```python
from build123d import *

# Parameters (mm, degrees)
SKETCH_1_W          = 300
SKETCH_1_H          = 300
EXTRUDE_1_DEPTH     = 5
SKETCH_2_R          = 1.6
CUT_EXTRUDE_1_DEPTH = 5
SKETCH_3_W          = 20
SKETCH_3_H          = 50
EXTRUDE_2_DEPTH     = 5
SKETCH_5_R          = 1.6
CUT_EXTRUDE_2_DEPTH = 462.004338374
CHAMFER_1_SIZE      = 20
FILLET_1_R          = 20
FILLET_2_R          = 5
FILLET_3_R          = 10


with BuildPart() as part:
    # 草图1 → 凸台-拉伸1 (new body)
    with BuildSketch(Plane.XY):
        with Locations((150, 150)):
            Rectangle(SKETCH_1_W, SKETCH_1_H)
    extrude(amount=EXTRUDE_1_DEPTH)

    # 草图2 → 切除-拉伸1 (cut)
    with BuildSketch(Plane.XY.offset(5)):
        with Locations((10, 10)):
            Circle(SKETCH_2_R)
        with Locations((290, 10)):
            Circle(SKETCH_2_R)
        with Locations((290, 290)):
            Circle(SKETCH_2_R)
        with Locations((10, 290)):
            Circle(SKETCH_2_R)
        with Locations((10, 270)):
            Circle(SKETCH_2_R)
        with Locations((10, 250)):
            Circle(SKETCH_2_R)
        with Locations((10, 30)):
            Circle(SKETCH_2_R)
        with Locations((10, 50)):
            Circle(SKETCH_2_R)
        with Locations((30, 290)):
            Circle(SKETCH_2_R)
        with Locations((50, 290)):
            Circle(SKETCH_2_R)
        with Locations((270, 290)):
            Circle(SKETCH_2_R)
        with Locations((250, 290)):
            Circle(SKETCH_2_R)
        with Locations((290, 270)):
            Circle(SKETCH_2_R)
        with Locations((290, 250)):
            Circle(SKETCH_2_R)
        with Locations((290, 30)):
            Circle(SKETCH_2_R)
        with Locations((290, 50)):
            Circle(SKETCH_2_R)
        with Locations((270, 10)):
            Circle(SKETCH_2_R)
        with Locations((250, 10)):
            Circle(SKETCH_2_R)
        with Locations((30, 10)):
            Circle(SKETCH_2_R)
        with Locations((50, 10)):
            Circle(SKETCH_2_R)
    extrude(amount=-CUT_EXTRUDE_1_DEPTH, mode=Mode.SUBTRACT)

    # 草图3 → 凸台-拉伸2 (add, through all)
    with BuildSketch(Plane.XY.offset(5)):
        with Locations((80, -25)):
            Rectangle(SKETCH_3_W, SKETCH_3_H)
        with Locations((80, 325)):
            Rectangle(SKETCH_3_W, SKETCH_3_H)
        with Locations((220, 325)):
            Rectangle(SKETCH_3_W, SKETCH_3_H)
        with Locations((220, -25)):
            Rectangle(SKETCH_3_W, SKETCH_3_H)
    extrude(amount=-EXTRUDE_2_DEPTH)

    # 草图5 → 切除-拉伸2 (cut, through all)
    with BuildSketch(Plane.XY.offset(5)):
        with Locations((80, 345)):
            Circle(SKETCH_5_R)
        with Locations((80, 325)):
            Circle(SKETCH_5_R)
        with Locations((80, 305)):
            Circle(SKETCH_5_R)
        with Locations((80, 255)):
            Circle(SKETCH_5_R)
        with Locations((80, 275)):
            Circle(SKETCH_5_R)
        with Locations(Location((80, 25, 0), (0, 0, 180))):
            Circle(SKETCH_5_R)
        with Locations(Location((80, 45, 0), (0, 0, 180))):
            Circle(SKETCH_5_R)
        with Locations(Location((80, -5, 0), (0, 0, 180))):
            Circle(SKETCH_5_R)
        with Locations(Location((80, -25, 0), (0, 0, 180))):
            Circle(SKETCH_5_R)
        with Locations(Location((80, -45, 0), (0, 0, 180))):
            Circle(SKETCH_5_R)
        with Locations((220, -45)):
            Circle(SKETCH_5_R)
        with Locations((220, -25)):
            Circle(SKETCH_5_R)
        with Locations((220, -5)):
            Circle(SKETCH_5_R)
        with Locations((220, 45)):
            Circle(SKETCH_5_R)
        with Locations((220, 25)):
            Circle(SKETCH_5_R)
        with Locations(Location((220, 275, 0), (0, 0, 180))):
            Circle(SKETCH_5_R)
        with Locations(Location((220, 255, 0), (0, 0, 180))):
            Circle(SKETCH_5_R)
        with Locations(Location((220, 305, 0), (0, 0, 180))):
            Circle(SKETCH_5_R)
        with Locations(Location((220, 325, 0), (0, 0, 180))):
            Circle(SKETCH_5_R)
        with Locations(Location((220, 345, 0), (0, 0, 180))):
            Circle(SKETCH_5_R)
    extrude(amount=-CUT_EXTRUDE_2_DEPTH, mode=Mode.SUBTRACT)

    # 倒角1
    chamfer_1_edges = [part.edges().sort_by_distance(p)[0] for p in [
        (210, 0, 2.5),
        (230, 0, 2.5),
        (230, 300, 2.5),
        (210, 300, 2.5),
        (90, 300, 2.5),
        (70, 300, 2.5),
        (70, 0, 2.5),
        (90, 0, 2.5),
    ]]
    chamfer(chamfer_1_edges, length=CHAMFER_1_SIZE)

    # 圆角1
    fillet_1_edges = [part.edges().sort_by_distance(p)[0] for p in [
        (230, -20, 2.5),
        (250, 0, 2.5),
        (110, 0, 2.5),
        (190, 0, 2.5),
        (210, -20, 2.5),
        (90, -20, 2.5),
        (50, 0, 2.5),
        (70, -20, 2.5),
        (250, 300, 2.5),
        (230, 320, 2.5),
        (210, 320, 2.5),
        (110, 300, 2.5),
        (190, 300, 2.5),
        (90, 320, 2.5),
        (70, 320, 2.5),
        (50, 300, 2.5),
    ]]
    fillet(fillet_1_edges, radius=FILLET_1_R)

    # 圆角2
    fillet_2_edges = [part.edges().sort_by_distance(p)[0] for p in [
        (230, -50, 2.5),
        (210, -50, 2.5),
        (230, 350, 2.5),
        (210, 350, 2.5),
        (70, 350, 2.5),
        (90, 350, 2.5),
        (70, -50, 2.5),
        (90, -50, 2.5),
    ]]
    fillet(fillet_2_edges, radius=FILLET_2_R)

    # 圆角3
    fillet_3_edges = [part.edges().sort_by_distance(p)[0] for p in [
        (0, 300, 2.5),
        (300, 300, 2.5),
        (300, 0, 2.5),
        (0, 0, 2.5),
    ]]
    fillet(fillet_3_edges, radius=FILLET_3_R)


solid = part.part
```
Check sheet for the modelled part. Datum: model origin and axes. Units: mm. A direction names the side the tool comes from. Round coordinates to 2 decimals unless told otherwise and drop trailing zeros. Order: outer loops, then holes, each group sorted by start corner. A loop starts at its lowest first (then second) coordinate and runs counter-clockwise, first axis right, second up.
1) Mould release check, pull along X, two halves, no side actions. Record for faces 1 (the flat face through (240, 310, 3)), 2 (the flat face through (60, 310, 3)), 3 (the flat face through (100, -10, 3)): +X half, -X half, draft (parallel to the pull), parting line (faces both ways), or undercut.
2) Section check A-A (z = 2.05). Give the number of separate pieces and of enclosed holes in the cut face, and give its area (3 significant figures).
3) Go/stop test with flat-tipped pins: pin 1 Ø2.5 at (x, y) = (220, 305) entering from +Z; pin 2 Ø3 at (x, z) = (207, 2) entering from +Y. Record where each tip stops, or that it passes through.
4) Scan lines: line 1 (Y direction, x = 174, z = 1.9); line 2 (X direction, y = -18, z = 0.8); line 3 (X direction, y = 7.5, z = 2.45). Record each from-to range of solid material in increasing order.
5) Section check B-B (x = 143.5). Record the boundary of the cut face in (y, z), and give its area (3 significant figures).
6) Tool access check on faces 4 (the flat face through (200, -10, 3)), 5 (the flat face through (60, -10, 3)), 6 (the flat face through (100, 310, 3)). Record the directions out of +Z, -Z, +X, -X, +Y, -Y that give a thin tool (end or side, any length) a straight path to the whole face; none if there is none.
Result:
1. face 1: +X half
1. face 2: -X half
1. face 3: undercut
2. separate pieces: 1
2. enclosed holes: 40
2. area: 95,300 mm2
3. pin 1: passes through
3. pin 2: stops at y = 320.68
4. line 1: y = 0 to 300
4. line 2: x = 67.15 to 92.85, 207.15 to 232.85
4. line 3: x = 0.32 to 299.68
5. outline: (0, 0) - (300, 0) - (300, 5) - (0, 5) - close
5. area: 1,500 mm2
6. face 4: +Z, -Z, -Y
6. face 5: +Z, -Z, -X, -Y
6. face 6: +Z, -Z, +Y
